Autodesk Inventor part; units mm, degrees
ref_plane "YZ Plane" through (0, 0, 0) normal (1, 0, 0) x (0, 1, 0)
ref_plane "XZ Plane" through (0, 0, 0) normal (0, 1, 0) x (-1, 0, 0)
ref_plane "XY Plane" through (0, 0, 0) normal (0, 0, 1) x (1, 0, 0)
sketch "Sketch1" plane through (0, 0, 0) normal (0, 0, 1) x (1, 0, 0)
  point P0 (0, 0)
sketch "Sketch2" plane through (0, 0, 0) normal (0, 0, 1) x (1, 0, 0)
  circle A0 centre (0, 0) radius 3
  circle A1 centre (78, 0) radius 3
  arc A2 (0, 4) -> (0, -4) centre (0, 0) ccw
  arc A3 (78, -4) -> (78, 4) centre (78, 0) ccw
  line L0 (0, 4) -> (78, 4)
  line L1 (78, -4) -> (0, -4)
  dimension "d0" = 6
  dimension "d1" = 6
  dimension "d2" = 78
  dimension "d3" = 8
  dimension "d4" = 8
extrude "Extrusion1" add sketch "Sketch2" along normal blind 10.2
properties part number "Connector to rod"
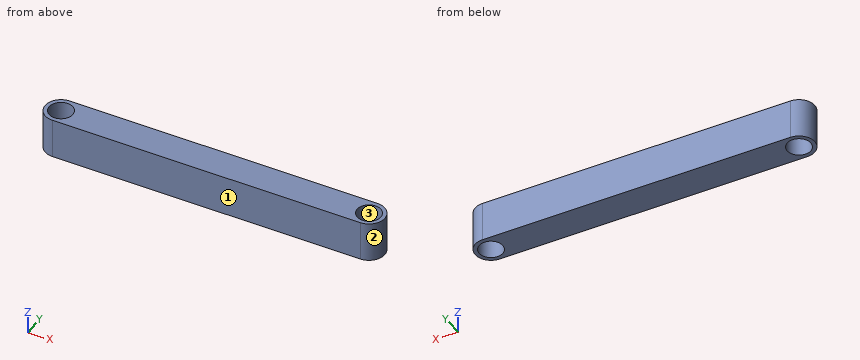
Check sheet for the modelled part. Datum: model origin and axes. Units: mm. Face numbers are marked on the shaded views. Round coordinates to 2 decimals unless told otherwise and drop trailing zeros. Loops run counter-clockwise (first coordinate to the right, second up) from the corner with the lowest first, then second, coordinate; pieces in that order, holes last. Notation, with made-up numbers: (-37.5, 64.5) - (15.5, 64.5) arc R26 cw to (15.5, 103.5) - close; hole circle Ø6 at (-6, 67.25). An arc over 180 degrees is marked (long way). Write item = value, one per line. Start each with the question number.
Q1. Release check for a two-part mould opening along X. For the marked faces 1, 2 and 3 record: pulls with the +X half, pulls with the -X half, needs draft (parallel to the pull), parting line crosses it, or undercut.
Q2. Section check B-B (z = 2). Record the boundary of the cut face in (x, y).
Q3. Depth check by flat-ended pin: P1, Ø1.5, axis at y = -1.5, z = 8.5, coming from the -X side. Enter the tip coordinate at first touch or a pass-through.
Q4. Thickness scan on L1, parallel to Y at x = 78, z = 6.5; L2, parallel to X at y = -2.75, z = 2.75; L3, parallel to X at y = 1.75, z = 4.5. Record the ranges inside material, lowest first.
Q5. Section check A-A (y = 0). Record the boundary of the cut face in (x, z).
Derived:
q1.face_1 = needs draft
q1.face_2 = pulls with the +X half
q1.face_3 = undercut
q2.outline = (0, -4) - (78, -4) arc R4 ccw to (78, 4) - (0, 4) arc R4 ccw to start; hole circle Ø6 at (0, 0); hole circle Ø6 at (78, 0)
q3.P1 = -3.93
q4.L1 = -4 to -3, 3 to 4
q4.L2 = -2.9 to -1.2, 1.2 to 76.8, 79.2 to 80.9
q4.L3 = -3.6 to -2.44, 2.44 to 75.56, 80.44 to 81.6
q5.outline = (-4, 0) - (-3, 0) - (-3, 10.2) - (-4, 10.2) - close; (3, 0) - (75, 0) - (75, 10.2) - (3, 10.2) - close; (81, 0) - (82, 0) - (82, 10.2) - (81, 10.2) - close
